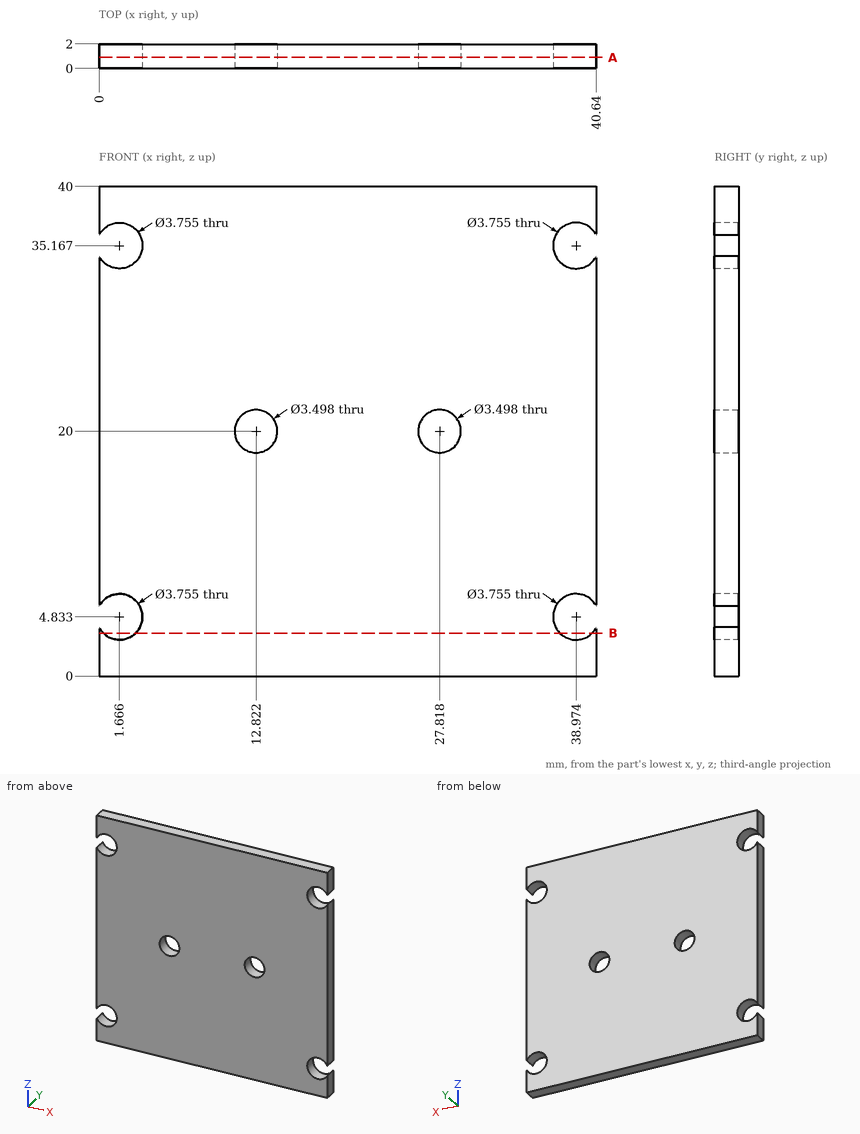
Print and shaded views of the part. All mm, measured from the part's lowest x, y and z. Round coordinates to 2 decimals unless told otherwise and drop trailing zeros. Loops run counter-clockwise (first coordinate to the right, second up) from the corner with the lowest first, then second, coordinate; pieces in that order, holes last. Notation, with made-up numbers: M 67.25,-25.75 L 89.25,-25.75 A18 cw 89.25,-12.75 Z; hole C 42.5,-14.75 d5. An arc over 180 degrees is marked long. One line per question, with ' | ' between items.
1) Flat gauge pin, fed straight in: pin 1 (3 mm diameter, centred on x = 1.67, z = 35.17, fed in from -Y). Where does the tip first touch, or does it go through?
Solved:
pin 1: passes through
2) Band-saw the part on A-A (y = 0.9). Give the number of separate pieces and of enclosed holes in the cut face, then the cut area to 3 significant figures.
Solved:
separate pieces: 1 | enclosed holes: 2 | area: 1,560 mm²
3) Band-saw the part on B-B (z = 3.5). Give the cut face in (x, y).
Solved:
outline: M 0,0 L 0.34,0 L 0.34,2 L 0,2 Z; M 2.99,0 L 37.65,0 L 37.65,2 L 2.99,2 Z; M 40.3,0 L 40.64,0 L 40.64,2 L 40.3,2 Z
4) Drill centre lines: line 1 along X through (y, z) = (1, 5) (1 decimal); line 2 along Z through (x, y) = (37.5, 0.35) (1 decimal); line 3 along X through (y, z) = (1, 34.5). Where is each one in solid material? Low to high.
Solved:
line 1: x = 3.5 to 37.1 | line 2: z = 0 to 3.7, 6 to 34, 36.3 to 40 | line 3: x = 3.42 to 37.22
